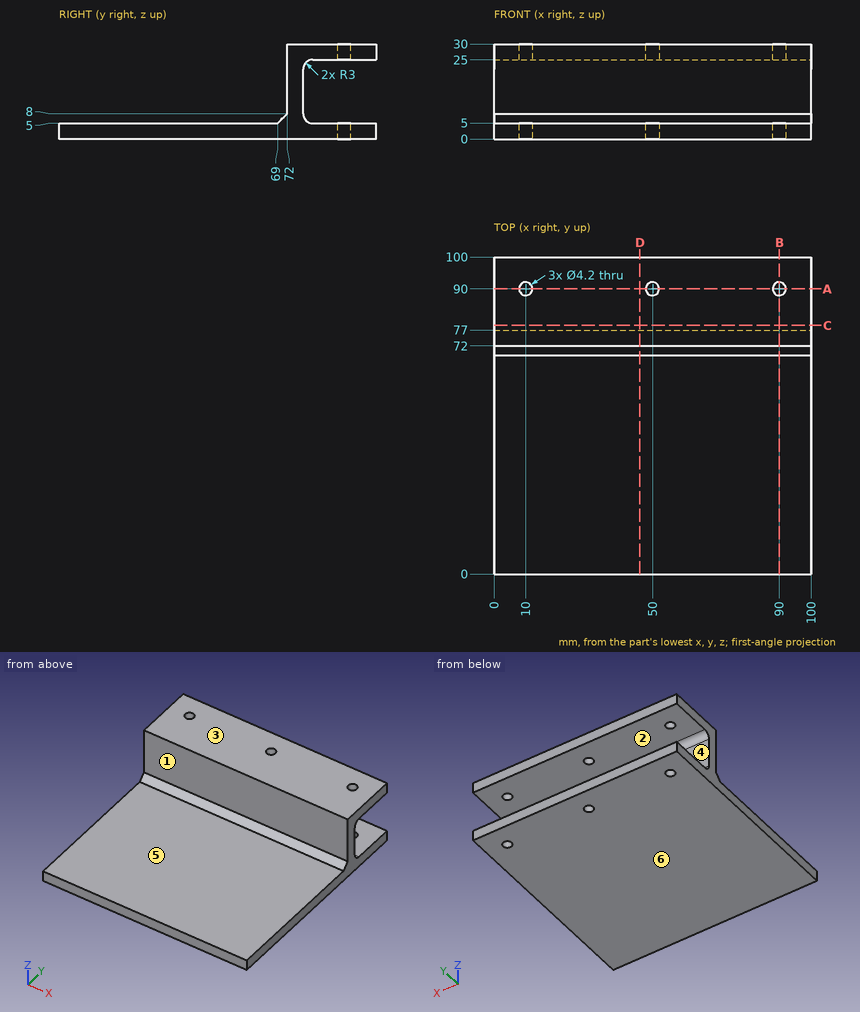
Source: three-view drawing plus pictorial views. Frame: mm from the lowest corner of the part. A direction names the side the tool comes from. Coordinates: 2 decimals unless noted, no trailing zeros. Write each loop counter-clockwise with the first axis right and the second up, starting at its lowest first coordinate (ties: lowest second). Pieces come first, ordered by that corner, then holes. Notation, with made-up numbers: (-13, 56.5) - (9, 56.5) arc R10 cw to (9, 69.5) - close; hole circle Ø2 at (78.5, 66). An arc over 180 degrees is marked (long way). Answer as a JSON object with one key per item and string values.
Q1. Section query C-C, the plane y = 78.5. Output: boundary loops of the cut face in (x, z), plus the area to 3 significant figures.
Ans:
{"outline": "(0, 0) - (100, 0) - (100, 5.4) - (0, 5.4) - close; (0, 24.6) - (100, 24.6) - (100, 30) - (0, 30) - close", "area": "1,080 mm2"}
Q2. Material intervals for line 1 (X direction, y = 90, z = 28.65); line 2 (Y direction, x = 10, z = 27.9); line 3 (Z direction, x = 36.5, y = 89.5), sorted ascending. Write a range as [from, to].
Ans:
{"line 1": "x = [0, 7.9], [12.1, 47.9], [52.1, 87.9], [92.1, 100]", "line 2": "y = [72, 87.9], [92.1, 100]", "line 3": "z = [0, 5], [25, 30]"}
Q3. Draft query along Z for the marked faces 4, 5 and 6. Return one class per face: released by +Z, released by -Z, zero draft, split by the parting line, or undercut.
Ans:
{"face 4": "undercut", "face 5": "released by +Z", "face 6": "released by -Z"}
Q4. Set-up query: the marked faces 1, 2 and 3. Return all of +Z, -Z, +X, -X, +Y, -Y with unobstructed straight access to the full face (end or side cutting, diameter ignored); none if empty.
Ans:
{"face 1": "+Z, +X, -X, -Y", "face 2": "+X, -X, +Y", "face 3": "+Z, +X, -X, +Y, -Y"}
Q5. First-contact query: pin 1 Ø8 at (y, z) = (79.5, 23) entering from +X; pin 2 Ø2 at (x, z) = (33.5, 24.5) entering from -Y; pin 3 Ø11 at (x, z) = (55, 14.5) entering from +Y. Flat tips, straight axial feed; report the tip coordinate or a pass-through.
Ans:
{"pin 1": "stops at x = 100", "pin 2": "stops at y = 72", "pin 3": "stops at y = 77"}
Q6. Section query A-A, the plane y = 90. State how many separate pieces and enclosed holes the cut face has, plus the area to 3 significant figures.
Ans:
{"separate pieces": "8", "enclosed holes": "0", "area": "874 mm2"}
Q7. Section query B-B, the plane x = 90. Output: boundary loops of the cut face in (y, z), plus the area to 3 significant figures.
Ans:
{"outline": "(0, 0) - (87.9, 0) - (87.9, 5) - (80, 5) arc R3 cw to (77, 8) - (77, 22) arc R3 cw to (80, 25) - (87.9, 25) - (87.9, 30) - (72, 30) - (72, 8) - (69, 5) - (0, 5) - close; (92.1, 0) - (100, 0) - (100, 5) - (92.1, 5) - close; (92.1, 25) - (100, 25) - (100, 30) - (92.1, 30) - close", "area": "706 mm2"}
Q8. Section query D-D, the plane x = 46. Output: boundary loops of the cut face in (y, z), plus the area to 3 significant figures.
Ans:
{"outline": "(0, 0) - (100, 0) - (100, 5) - (80, 5) arc R3 cw to (77, 8) - (77, 22) arc R3 cw to (80, 25) - (100, 25) - (100, 30) - (72, 30) - (72, 8) - (69, 5) - (0, 5) - close", "area": "748 mm2"}
